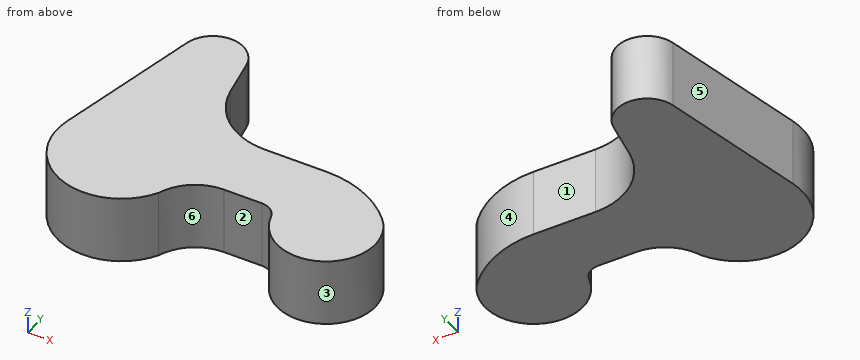
from build123d import *

# Parameters (mm, degrees)
F1_DEPTH = 40


with BuildPart() as f1:
    # F0 (on Top) → F1 (new body)
    with BuildSketch(Plane.XY):
        with BuildLine():
            Line((-17.559889, 94.956044), (-37.070878, 8.351648))
            ThreePointArc((-37.070878, 8.351648), (-13.833241, -35.392675), (32.908965, -19))
            ThreePointArc((32.908965, -19), (43.455181, -5.223464), (60, 0))
            Line((60, 0), (82.303846, 0))
            ThreePointArc((82.303846, 0), (88.401345, -2.074061), (91.969527, -7.435897))
            ThreePointArc((91.969527, -7.435897), (133.948558, -25.42514), (141.332314, 19.645161))
            ThreePointArc((141.332314, 19.645161), (121.293071, 33.948656), (97.196491, 39))
            Line((97.196491, 39), (61, 39))
            ThreePointArc((61, 39), (35.28131, 48.364253), (21.604436, 72.072551))
            Line((21.604436, 72.072551), (17.728004, 94.117352))
            ThreePointArc((17.728004, 94.117352), (0.427687, 108.994918), (-17.559889, 94.956044))
        make_face()
    extrude(amount=F1_DEPTH)


solid = f1.part
Geometry check sheet. Reference: the model listing, model coordinates, mm. Face numbers are marked on the shaded views. A direction names the side the tool comes from. Round coordinates to 2 decimals unless told otherwise and drop trailing zeros. Write each loop counter-clockwise with the first axis right and the second up, starting at its lowest first coordinate (ties: lowest second). Pieces come first, ordered by that corner, then holes. Notation, with made-up numbers: (48, -13) - (75, -13) arc R26 cw to (75, 7) - close; hole circle Ø5 at (43, 25). An arc over 180 degrees is marked (long way). One line per item, written item: value.
1. Cross-section at A-A on z = 9.5. Record the boundary of the cut face in (x, y).
The answers:
outline: (-37.07, 8.35) arc R38 ccw to (32.91, -19) arc R28.81 cw to (60, 0) - (82.3, 0) arc R10 cw to (91.97, -7.44) arc R29 ccw (long way) to (141.33, 19.65) arc R60 ccw to (97.2, 39) - (61, 39) arc R40 cw to (21.6, 72.07) - (17.73, 94.12) arc R18 ccw to (-17.56, 94.96) - close
2. Cross-section at B-B on x = 74.5. Record the boundary of the cut face in (y, z).
The answers:
outline: (0, 0) - (39, 0) - (39, 40) - (0, 40) - close
3. Scan lines: L1, parallel to X at y = -3, z = 28; L2, parallel to Y at x = 62.5, z = 8.5; L3, parallel to X at y = -20, z = 18.5. Record each from-to range of solid material in increasing order.
The answers:
L1: x = -37.88 to 47.2, 89.45 to 148.84
L2: y = 0 to 39
L3: x = -32.31 to 32.31, 99 to 141
4. Cross-section at C-C on y = 85. Record the boundary of the cut face in (x, z), and give its area (3 significant figures).
The answers:
outline: (-19.8, 0) - (19.33, 0) - (19.33, 40) - (-19.8, 40) - close
area: 1,570 mm^2
5. Depth check by flat-ended pin: pin 1 Ø2 at (y, z) = (88.5, 34.5) entering from -X; pin 2 Ø2 at (y, z) = (32, 24) entering from +X; pin 3 Ø5 at (x, z) = (61, 24) entering from -Y. Enter the tip coordinate at first touch or a pass-through.
The answers:
pin 1: stops at x = -19.24
pin 2: stops at x = 127.13
pin 3: stops at y = -0.04
6. Set-up check for the marked faces 1, 2 and 3: record each of +Z, -Z, +X, -X, +Y, -Y from which the full face is reachable in a straight line by a thin tool's end or side.
The answers:
face 1: +Z, -Z, +X, +Y
face 2: +Z, -Z, -Y
face 3: +Z, -Z
7. Mould release check, pull along X, two halves, no side actions. Record for the marked faces 4, 5 and 6: released by +X, released by -X, zero draft, split by the parting line, or undercut.
The answers:
face 4: released by +X
face 5: released by -X
face 6: undercut
